Verification items for the finished model (mm, model axes). Face numbers are marked on the shaded views. A direction names the side the tool comes from. Give positions to 0.01 mm unless a question says otherwise; leave off trailing zeros. Order: outer loops, then holes, each group sorted by start corner. A loop starts at its lowest first (then second) coordinate and runs counter-clockwise, first axis right, second up. Notation, with made-up numbers: M 61,-28 L 103,-28 A21 cw 103,8 Z; hole C 89.25,-27 d11. An arc over 180 degrees is marked long. Answer as a JSON object with one key per item and string values.
```python
from build123d import *

# Parameters (mm, degrees)
SKETCH1_W                    = 66.675
SKETCH1_H                    = 31.75
BOSS_EXTRUDE1_DEPTH          = 23.495
CUT_EXTRUDE1_REACH           = 61.762
SKETCH2_W                    = 47.625
SKETCH2_H                    = 23.550328578
CUT_EXTRUDE2_REACH           = 53.686
SKETCH3_W                    = 47.625
SKETCH3_H                    = 19.05
F_1_4_20_TAPPED_HOLE1_REACH  = 74.454
F_1_4_20_TAPPED_HOLE1_BORE_R = 2.5527
F_8_32_TAPPED_HOLE1_D        = 3.4544
F_8_32_TAPPED_HOLE1_DEPTH    = 12.446
F_8_32_TAPPED_HOLE1_TIP      = 1.037806461
F_6_32_TAPPED_HOLE1_D        = 2.7051
F_6_32_TAPPED_HOLE1_DEPTH    = 13.716
F_6_32_TAPPED_HOLE1_TIP      = 0.81269403


with BuildPart() as part:
    # Sketch1 → Boss-Extrude1 (new, symmetric)
    with BuildSketch(Plane(origin=(0, 0, 0), x_dir=(1, 0, 0), z_dir=(0, 1, 0))):
        Rectangle(SKETCH1_W, SKETCH1_H)
    extrude(amount=BOSS_EXTRUDE1_DEPTH, both=True)

    # Sketch2 → Cut-Extrude1 (cut, up to next)
    with BuildSketch(Plane(origin=(0, 23.495, 0), x_dir=(1, 0, 0), z_dir=(0, 1, 0)), mode=Mode.PRIVATE) as cut_extrude1_sk1:
        with Locations((0, -4.099835711)):
            Rectangle(SKETCH2_W, SKETCH2_H)
    cut_extrude1_tool1 = extrude(cut_extrude1_sk1.sketch, amount=-CUT_EXTRUDE1_REACH, mode=Mode.PRIVATE) & part.part
    add(cut_extrude1_tool1.solids().sort_by_distance((0, 23.495, 4.099836))[0], mode=Mode.SUBTRACT)

    # Sketch3 → Cut-Extrude2 (cut, up to next)
    with BuildSketch(Plane(origin=(0, 0, -15.875), x_dir=(-1, 0, 0), z_dir=(0, 0, -1)), mode=Mode.PRIVATE) as cut_extrude2_sk1:
        with Locations((0, -13.97)):
            Rectangle(SKETCH3_W, SKETCH3_H)
    cut_extrude2_tool1 = extrude(cut_extrude2_sk1.sketch, amount=-CUT_EXTRUDE2_REACH, mode=Mode.PRIVATE) & part.part
    add(cut_extrude2_tool1.solids().sort_by_distance((0, -13.97, -15.875))[0], mode=Mode.SUBTRACT)

    # 1_4-20 Tapped Hole1 bore → 1_4-20 Tapped Hole1 (cut, up to next)
    with BuildSketch(Plane(origin=(33.3375, 0, 0), x_dir=(0, 0, -1), z_dir=(1, 0, 0)), mode=Mode.PRIVATE) as f_1_4_20_tapped_hole1_sk1:
        with Locations((-9.525, 15.875)):
            Circle(F_1_4_20_TAPPED_HOLE1_BORE_R)
    f_1_4_20_tapped_hole1_tool1 = extrude(f_1_4_20_tapped_hole1_sk1.sketch, amount=-F_1_4_20_TAPPED_HOLE1_REACH, mode=Mode.PRIVATE) & part.part
    # 1_4-20 Tapped Hole1 bore → 1_4-20 Tapped Hole1 (cut, up to next)
    with BuildSketch(Plane(origin=(33.3375, 0, 0), x_dir=(0, 0, -1), z_dir=(1, 0, 0)), mode=Mode.PRIVATE) as f_1_4_20_tapped_hole1_sk2:
        with Locations((3.175, 15.875)):
            Circle(F_1_4_20_TAPPED_HOLE1_BORE_R)
    f_1_4_20_tapped_hole1_tool2 = extrude(f_1_4_20_tapped_hole1_sk2.sketch, amount=-F_1_4_20_TAPPED_HOLE1_REACH, mode=Mode.PRIVATE) & part.part
    # 1_4-20 Tapped Hole1 bore → 1_4-20 Tapped Hole1 (cut, up to next)
    with BuildSketch(Plane(origin=(33.3375, 0, 0), x_dir=(0, 0, -1), z_dir=(1, 0, 0)), mode=Mode.PRIVATE) as f_1_4_20_tapped_hole1_sk3:
        with Locations((3.175, -3.175)):
            Circle(F_1_4_20_TAPPED_HOLE1_BORE_R)
    f_1_4_20_tapped_hole1_tool3 = extrude(f_1_4_20_tapped_hole1_sk3.sketch, amount=-F_1_4_20_TAPPED_HOLE1_REACH, mode=Mode.PRIVATE) & part.part
    # 1_4-20 Tapped Hole1 bore → 1_4-20 Tapped Hole1 (cut, up to next)
    with BuildSketch(Plane(origin=(33.3375, 0, 0), x_dir=(0, 0, -1), z_dir=(1, 0, 0)), mode=Mode.PRIVATE) as f_1_4_20_tapped_hole1_sk4:
        with Locations((-9.525, -3.175)):
            Circle(F_1_4_20_TAPPED_HOLE1_BORE_R)
    f_1_4_20_tapped_hole1_tool4 = extrude(f_1_4_20_tapped_hole1_sk4.sketch, amount=-F_1_4_20_TAPPED_HOLE1_REACH, mode=Mode.PRIVATE) & part.part
    f_1_4_20_tapped_hole1_1 = f_1_4_20_tapped_hole1_tool1.solids().sort_by_distance((33.3375, 15.875, 9.525))[0]
    add(f_1_4_20_tapped_hole1_1, mode=Mode.SUBTRACT)
    f_1_4_20_tapped_hole1_2 = f_1_4_20_tapped_hole1_tool2.solids().sort_by_distance((33.3375, 15.875, -3.175))[0]
    add(f_1_4_20_tapped_hole1_2, mode=Mode.SUBTRACT)
    f_1_4_20_tapped_hole1_3 = f_1_4_20_tapped_hole1_tool3.solids().sort_by_distance((33.3375, -3.175, -3.175))[0]
    add(f_1_4_20_tapped_hole1_3, mode=Mode.SUBTRACT)
    f_1_4_20_tapped_hole1_4 = f_1_4_20_tapped_hole1_tool4.solids().sort_by_distance((33.3375, -3.175, 9.525))[0]
    add(f_1_4_20_tapped_hole1_4, mode=Mode.SUBTRACT)
    f_1_4_20_tapped_hole1 = f_1_4_20_tapped_hole1_1 + f_1_4_20_tapped_hole1_2 + f_1_4_20_tapped_hole1_3 + f_1_4_20_tapped_hole1_4  # 1_4-20 Tapped Hole1 as one shape, for the pattern or mirror that repeats it

    # Mirror1: 1_4-20 Tapped Hole1 across plane
    add(f_1_4_20_tapped_hole1.mirror(Plane(origin=(0, 0, 0), x_dir=(0, 0, 1), z_dir=(1, 0, 0))), mode=Mode.SUBTRACT)

    # 8-32 Tapped Hole1
    with Locations(Plane.XY.offset(15.875)):
        with Locations((-26.9875, -12.065), (26.9875, -12.065)):
            Hole(F_8_32_TAPPED_HOLE1_D / 2, depth=F_8_32_TAPPED_HOLE1_DEPTH)
            with Locations((0, 0, -(F_8_32_TAPPED_HOLE1_DEPTH + F_8_32_TAPPED_HOLE1_TIP / 2))):  # 118° drill point
                Cone(0, F_8_32_TAPPED_HOLE1_D / 2, F_8_32_TAPPED_HOLE1_TIP, mode=Mode.SUBTRACT)

    # 6-32 Tapped Hole1
    with Locations(Plane(origin=(0, 23.495, 0), x_dir=(1, 0, 0), z_dir=(0, 1, 0))):
        with Locations((0, 11.811), (19.05, 11.811), (-19.05, 11.811), (-28.575, -3.175), (28.575, -3.175)):
            Hole(F_6_32_TAPPED_HOLE1_D / 2, depth=F_6_32_TAPPED_HOLE1_DEPTH)
            with Locations((0, 0, -(F_6_32_TAPPED_HOLE1_DEPTH + F_6_32_TAPPED_HOLE1_TIP / 2))):  # 118° drill point
                Cone(0, F_6_32_TAPPED_HOLE1_D / 2, F_6_32_TAPPED_HOLE1_TIP, mode=Mode.SUBTRACT)


solid = part.part
```
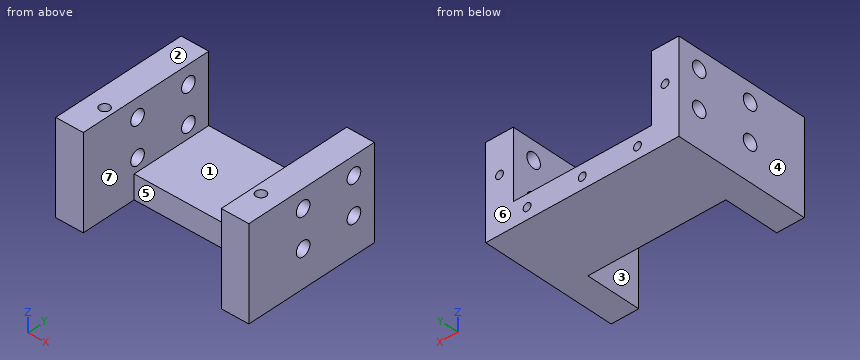
Q1. Release check for a two-part mould opening along X. For the marked faces 1, 2, 3 and 4 record: +X half, -X half, draft (parallel to the pull), parting line (faces both ways), or undercut.
Resolved:
{"face 1": "undercut", "face 2": "draft", "face 3": "undercut", "face 4": "-X half"}
Q2. Section check C-C on y = -18. Record the cut outline in (x, z) (1 decimal), then the cut area to 3 significant figures.
Resolved:
{"outline": "M -33.3,-15.9 L -23.8,-15.9 L -23.8,15.9 L -33.3,15.9 Z; M 23.8,-15.9 L 33.3,-15.9 L 33.3,15.9 L 23.8,15.9 Z", "area": "605 mm²"}
Q3. Gauge pin test, flat ends, axial feed: pin 1 Ø1.6 at (x, z) = (0, -11.811) entering from +Y; pin 2 Ø3.5 at (x, z) = (-19.05, -11.811) entering from +Y (3 decimals); pin 3 Ø14 at (x, y) = (-5.5, 16.5) entering from +Z; pin 4 Ø3 at (x, z) = (19.05, -11.811) entering from -Y (3 decimals). Record the tip position at first contact, or that the pin passes through.
Resolved:
{"pin 1": "stops at y = 9.45", "pin 2": "stops at y = 23.495", "pin 3": "stops at z = -7.68", "pin 4": "stops at y = -4.445"}
Q4. Tool access check on the marked faces 5, 6 and 7. Record the directions out of +Z, -Z, +X, -X, +Y, -Y that give a thin tool (end or side, any length) a straight path to the whole face; none if there is none.
Resolved:
{"face 5": "+Z, -Z, -Y", "face 6": "+Z, -Z, +X, -X, +Y", "face 7": "+Z, -Y"}
Q5. Section check A-A on y = 15. Count the separate pieces of the cut face and the enclosed holes in it, then the cut area to 3 significant figures.
Resolved:
{"separate pieces": "5", "enclosed holes": "5", "area": "784 mm²"}
Q6. Section check D-D on z = -9. Record the cut outline in (x, y) (1 decimal).
Resolved:
{"outline": "M -33.3,-23.5 L -23.8,-23.5 L -23.8,-4.4 L 23.8,-4.4 L 23.8,-23.5 L 33.3,-23.5 L 33.3,23.5 L -33.3,23.5 Z"}
Q7. Material ranges on L1, parallel to X at y = 3, z = 12.5; L2, parallel to X at y = 15.5, z = -13; L3, parallel to Z at x = 19, y = 15 (3 decimals), recorded low to high.
Resolved:
{"L1": "x = -33.34 to -23.81, 23.81 to 33.34", "L2": "x = -33.34 to -19.69, -18.41 to -0.64, 0.64 to 18.41, 19.69 to 33.34", "L3": "z = -15.875 to -13.163, -10.459 to -7.675"}
Q8. Section check B-B on z = 8.5. Record the cut outline in (x, y) (1 decimal), then the cut area to 3 significant figures.
Resolved:
{"outline": "M -33.3,-23.5 L -23.8,-23.5 L -23.8,-5.5 L -33.3,-5.5 Z; M -33.3,-0.8 L -23.8,-0.8 L -23.8,13.5 L -33.3,13.5 Z; M -33.3,18.2 L -23.8,18.2 L -23.8,23.5 L -33.3,23.5 Z; M 23.8,-23.5 L 33.3,-23.5 L 33.3,-5.5 L 23.8,-5.5 Z; M 23.8,-0.8 L 33.3,-0.8 L 33.3,13.5 L 23.8,13.5 Z; M 23.8,18.2 L 33.3,18.2 L 33.3,23.5 L 23.8,23.5 Z; hole C -27,-12.1 d3.5; hole C 27,-12.1 d3.5", "area": "698 mm²"}
